Source: CAD feature listing. Evaluate the final solid. Frame: model axes, mm. Give positions to 0.01 mm unless a question says otherwise; leave off trailing zeros. Order: outer loops, then holes, each group sorted by start corner. A loop starts at its lowest first (then second) coordinate and runs counter-clockwise, first axis right, second up. Notation, with made-up numbers: (79.5, 87) - (86.5, 87) arc R12 ccw to (86.5, 99) - close; hole circle Ø11 at (12.25, -25.75). An arc over 180 degrees is marked (long way). Use CSV: the item, a comma, the result in double quotes.
```python
from build123d import *

# Parameters (mm, degrees)
SKETCH1_W               = 180
SKETCH1_H               = 122.36
BOSS_EXTRUDE1_DEPTH     = 3.18
CUT_EXTRUDE1_DEPTH      = 1
CUT_EXTRUDE1_DEPTH_BACK = 4.18
SKETCH3_W               = 70.125
SKETCH3_H               = 3.18
SKETCH3_W_2             = 90.125
CUT_EXTRUDE2_DEPTH      = 1
CUT_EXTRUDE2_DEPTH_BACK = 4.18
SKETCH4_R               = 1.55
CUT_EXTRUDE3_DEPTH      = 1
CUT_EXTRUDE3_DEPTH_BACK = 4.18
SKETCH6_R               = 1.6
CUT_EXTRUDE4_DEPTH      = 1
CUT_EXTRUDE4_DEPTH_BACK = 4.18
SKETCH7_W               = 85
SKETCH7_H               = 55.6
CUT_EXTRUDE5_DEPTH      = 1
CUT_EXTRUDE5_DEPTH_BACK = 4.18
SKETCH8_W               = 80.125
SKETCH8_H               = 3.18
CUT_EXTRUDE6_DEPTH      = 1
CUT_EXTRUDE6_DEPTH_BACK = 4.18
SKETCH9_R               = 1.55
CUT_EXTRUDE7_DEPTH      = 1
CUT_EXTRUDE7_DEPTH_BACK = 4.18


with BuildPart() as part:
    # Sketch1 → Boss-Extrude1 (new body)
    with BuildSketch(Plane.XY):
        Rectangle(SKETCH1_W, SKETCH1_H)
    extrude(amount=BOSS_EXTRUDE1_DEPTH)

    # Sketch2 → Cut-Extrude1 (cut, two sides)
    with BuildSketch(Plane.XY.offset(3.18)) as cut_extrude1_sk:
        Polygon((80, 1.5), (77, 1.5), (77, -1.5), (80, -1.5), (80, -3.5), (82.82, -3.5), (82.82, -1.5), (86.82, -1.5), (86.82, -10), (90, -10), (90, 10), (86.82, 10), (86.82, 1.5), (82.82, 1.5), (82.82, 3.5), (80, 3.5), align=None)
    extrude(amount=CUT_EXTRUDE1_DEPTH, mode=Mode.SUBTRACT)
    extrude(cut_extrude1_sk.sketch, amount=-CUT_EXTRUDE1_DEPTH_BACK, mode=Mode.SUBTRACT)

    # Sketch3 → Cut-Extrude2 (cut, two sides)
    with BuildSketch(Plane.XY.offset(3.18)) as cut_extrude2_sk:
        with Locations((-54.9375, -59.59)):
            Rectangle(SKETCH3_W, SKETCH3_H)
        with Locations((44.9375, -59.59)):
            Rectangle(SKETCH3_W_2, SKETCH3_H)
    extrude(amount=CUT_EXTRUDE2_DEPTH, mode=Mode.SUBTRACT)
    extrude(cut_extrude2_sk.sketch, amount=-CUT_EXTRUDE2_DEPTH_BACK, mode=Mode.SUBTRACT)

    # Sketch4 → Cut-Extrude3 (cut, two sides)
    with BuildSketch(Plane.XY.offset(3.18)) as cut_extrude3_sk:
        with Locations((-10, -59.18)):
            Circle(SKETCH4_R)
    extrude(amount=CUT_EXTRUDE3_DEPTH, mode=Mode.SUBTRACT)
    extrude(cut_extrude3_sk.sketch, amount=-CUT_EXTRUDE3_DEPTH_BACK, mode=Mode.SUBTRACT)

    # Sketch6 → Cut-Extrude4 (cut, two sides)
    with BuildSketch(Plane.XY.offset(3.18)) as cut_extrude4_sk:
        with Locations((-64.946313591, 14.6)):
            Circle(SKETCH6_R)
        with Locations((-80.246313591, -36.2)):
            Circle(SKETCH6_R)
        with Locations((-31.946313591, -37.8)):
            Circle(SKETCH6_R)
        with Locations((-37.046313591, 14.6)):
            Circle(SKETCH6_R)
    extrude(amount=CUT_EXTRUDE4_DEPTH, mode=Mode.SUBTRACT)
    extrude(cut_extrude4_sk.sketch, amount=-CUT_EXTRUDE4_DEPTH_BACK, mode=Mode.SUBTRACT)

    # Sketch7 → Cut-Extrude5 (cut, two sides)
    with BuildSketch(Plane(origin=(0, 0, 0), x_dir=(-1, 0, 0), z_dir=(0, 0, -1))) as cut_extrude5_sk:
        with Locations((-22.5, -12.359811841)):
            Rectangle(SKETCH7_W, SKETCH7_H)
    extrude(amount=CUT_EXTRUDE5_DEPTH, mode=Mode.SUBTRACT)
    extrude(cut_extrude5_sk.sketch, amount=-CUT_EXTRUDE5_DEPTH_BACK, mode=Mode.SUBTRACT)

    # Sketch8 → Cut-Extrude6 (cut, two sides)
    with BuildSketch(Plane.XY.offset(3.18)) as cut_extrude6_sk:
        with Locations((-49.9375, 59.59)):
            Rectangle(SKETCH8_W, SKETCH8_H)
        with Locations((49.9375, 59.59)):
            Rectangle(SKETCH8_W, SKETCH8_H)
    extrude(amount=CUT_EXTRUDE6_DEPTH, mode=Mode.SUBTRACT)
    extrude(cut_extrude6_sk.sketch, amount=-CUT_EXTRUDE6_DEPTH_BACK, mode=Mode.SUBTRACT)

    # Sketch9 → Cut-Extrude7 (cut, two sides)
    with BuildSketch(Plane.XY.offset(3.18)) as cut_extrude7_sk:
        with Locations((0, 59.18)):
            Circle(SKETCH9_R)
    extrude(amount=CUT_EXTRUDE7_DEPTH, mode=Mode.SUBTRACT)
    extrude(cut_extrude7_sk.sketch, amount=-CUT_EXTRUDE7_DEPTH_BACK, mode=Mode.SUBTRACT)


solid = part.part
```
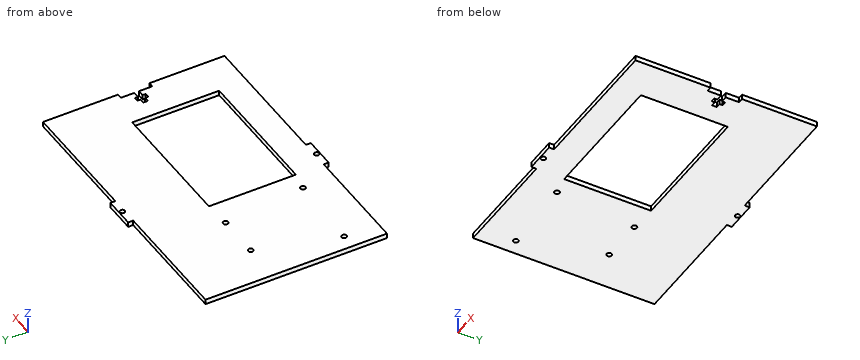
Item 1: Section C-C on z = 1.3. Count the separate pieces of the cut face and the enclosed holes in it, then the cut area to 3 significant figures.
Filled in:
separate pieces,"1"
enclosed holes,"7"
area,"16,100 mm2"
Item 2: Section D-D on x = -47.5. Return the cut outline in (y, z), then the cut area to 3 significant figures.
Filled in:
outline,"(-58, 0) - (58, 0) - (58, 3.18) - (-58, 3.18) - close"
area,"369 mm2"
Item 3: Material intervals for line 1 (Y direction, x = -10, z = 0.75); line 2 (Y direction, x = 0, z = 1.7); line 3 (Y direction, x = 3.5, z = 1.5), sorted ascending. Write a range as from..to.
Filled in:
line 1,"y = -61.18..-60.73, -57.63..-40.16, 15.44..58"
line 2,"y = -58..-40.16, 15.44..57.63, 60.73..61.18"
line 3,"y = -58..-40.16, 15.44..61.18"
Item 4: Section A-A on y = -12. Return the cut outline in (x, z).
Filled in:
outline,"(-90, 0) - (-20, 0) - (-20, 3.18) - (-90, 3.18) - close; (65, 0) - (90, 0) - (90, 3.18) - (65, 3.18) - close"
Item 5: First-contact query: pin 1 (1 mm diameter, centred on y = -5.5, z = 1.5, fed in from +X); pin 2 (0.9 mm diameter, centred on x = 79, z = 1, fed in from +Y); pin 3 (1 mm diameter, centred on y = -59, z = 1, fed in from -X) (3 decimals). Flat tips, straight axial feed; report the tip coordinate or a pass-through.
Filled in:
pin 1,"stops at x = 86.82"
pin 2,"stops at y = 58"
pin 3,"stops at x = -19.875"
Item 6: Section B-B on y = 7.5. Return the cut outline in (x, z), then the cut area to 3 significant figures.
Filled in:
outline,"(-90, 0) - (-20, 0) - (-20, 3.18) - (-90, 3.18) - close; (65, 0) - (86.82, 0) - (86.82, 3.18) - (65, 3.18) - close"
area,"292 mm2"
